Read the model definition and answer for the solid it produces. Units are mm, in the model's axes. A direction names the side the tool comes from. Coordinates: 2 decimals unless noted, no trailing zeros. Loops run counter-clockwise (first coordinate to the right, second up) from the corner with the lowest first, then second, coordinate; pieces in that order, holes last. Notation, with made-up numbers: (-9, 65.25) - (11, 65.25) arc R23 cw to (11, 81.25) - close; hole circle Ø7 at (71.5, 56.5). An arc over 180 degrees is marked (long way). Use one line per item in the form item = value.
from build123d import *


with BuildPart() as part:
    # 草图1 → 旋转1 (revolve)
    with BuildSketch(Plane(origin=(0, 0, 0), x_dir=(1, 0, 0), z_dir=(0, 1, 0)), mode=Mode.PRIVATE) as revolve_1_sk:
        Polygon((66, 7), (66, 8), (70, 8), (70, 21), (60, 21), (60, 11), (10, 11), (10, 21), (0, 21), (0, 8), (4, 8), (4, 7), align=None)
    revolve(revolve_1_sk.sketch.rotate(Axis((-74.515541445, 0, 0), (1, 0, 0)), 180), axis=Axis((-74.515541445, 0, 0), (1, 0, 0)))


solid = part.part
Item 1: The part is cut by section C-C on x = 5. Give the vertices of the cut face in (y, z), plus the area to 3 significant figures.
Results below:
outline = circle Ø42 at (0, 0); hole circle Ø14 at (0, 0)
area = 1,230 mm²
Item 2: For a pull along Y with two mould halves and no side action, classify faces 5 (the flat face through (10, 9, -9)), 6 (the cylindrical face through (64.93, -6.31, 20.03)), 7 (the flat face through (4, 6, 4)) as +Y half, -Y half, draft (parallel to the pull), parting line (faces both ways), or undercut.
Results below:
face_5 = draft
face_6 = parting line
face_7 = undercut
Item 3: Which of the six approach directions +Z, -Z, +X, -X, +Y, -Y give full straight-line access (tool end or side, diameter ignored) to faces 1 (the flat face through (60, 9, 9)), 2 (the flat face through (70, 0, -9)), 3 (the cylindrical face through (68.03, 7.81, -1.73)), 4 (the cylindrical face through (2.03, 7.81, -1.73))?
Results below:
face_1 = none
face_2 = +Z, -Z, +X, +Y, -Y
face_3 = +X
face_4 = -X
Item 4: The part is cut by section A-A on z = 0. Give the vertices of the cut face in (x, y).
Results below:
outline = (0, -21) - (10, -21) - (10, -11) - (60, -11) - (60, -21) - (70, -21) - (70, -8) - (66, -8) - (66, -7) - (4, -7) - (4, -8) - (0, -8) - close; (0, 8) - (4, 8) - (4, 7) - (66, 7) - (66, 8) - (70, 8) - (70, 21) - (60, 21) - (60, 11) - (10, 11) - (10, 21) - (0, 21) - close
Item 5: Find the intervals of material crossed by L1, parallel to X at y = 12, z = 15; L2, parallel to Y at x = 3.25, z = 0; L3, parallel to Z at x = 27, y = -4, in increasing order.
Results below:
L1 = 0 to 10, 60 to 70
L2 = -21 to -8, 8 to 21
L3 = -10.25 to -5.74, 5.74 to 10.25
Item 6: The part is cut by section D-D on z = 14.5. Give the vertices of the cut face in (x, y), plus the area to 3 significant figures.
Results below:
outline = (0, -15.19) - (10, -15.19) - (10, 15.19) - (0, 15.19) - close; (60, -15.19) - (70, -15.19) - (70, 15.19) - (60, 15.19) - close
area = 608 mm²
Item 7: Each of these flat-tipped pins is pushed along its axis until it touches: P1, Ø21, axis at y = -5.5, z = 1, coming from the -X side; P2, Ø6, axis at x = 37.5, z = -5.5, coming from the -Y side; P3, Ø1.5, axis at x = 9.5, y = -7, coming from the -Z side; P4, Ø10, axis at x = 20.5, y = 3, coming from the -Z side. Where does it stop, or does it pass through?
Results below:
P1 = 0
P2 = -10.71
P3 = -20.05
P4 = -11
